Geometry check sheet. Reference: the model listing, model coordinates, mm. Face numbers are marked on the shaded views. A direction names the side the tool comes from. Give positions to 0.01 mm unless a question says otherwise; leave off trailing zeros. Loops run counter-clockwise (first coordinate to the right, second up) from the corner with the lowest first, then second, coordinate; pieces in that order, holes last. Notation, with made-up numbers: (-11, -33) -> (25, -33) arc R13 cw to (25, -28) -> close; hole circle Ø4 at (9, 36). An arc over 180 degrees is marked (long way). Answer as a JSON object with one key per item and string values.
from build123d import *

# Parameters (mm, degrees)
SKETCH1_W           = 36
SKETCH1_H           = 48
BOSS_EXTRUDE1_DEPTH = 1.5
SKETCH1_3_R         = 13
BOSS_EXTRUDE2_DEPTH = 8.5
SKETCH1_4_W         = 13
SKETCH1_4_H         = 13
BOSS_EXTRUDE3_DEPTH = 12
SKETCH1_5_R         = 1.6
CUT_EXTRUDE2_DEPTH  = 33.310988843


with BuildPart() as part:
    # Sketch1 → Boss-Extrude1 (new body)
    with BuildSketch(Plane(origin=(0, 0, 0), x_dir=(1, 0, 0), z_dir=(0, 1, 0))):
        Rectangle(SKETCH1_W, SKETCH1_H)
    extrude(amount=BOSS_EXTRUDE1_DEPTH)

    # Sketch1_3 → Boss-Extrude2 (add)
    with BuildSketch(Plane(origin=(0, 0, 0), x_dir=(1, 0, 0), z_dir=(0, 1, 0))):
        with Locations(Location((0, 6, 0), (0, 0, 90))):
            Circle(SKETCH1_3_R)
    extrude(amount=BOSS_EXTRUDE2_DEPTH)

    # Sketch1_4 → Boss-Extrude3 (add)
    with BuildSketch(Plane(origin=(0, 0, 0), x_dir=(1, 0, 0), z_dir=(0, 1, 0))):
        with Locations((-10, -12.5)):
            Rectangle(SKETCH1_4_W, SKETCH1_4_H)
    extrude(amount=BOSS_EXTRUDE3_DEPTH)

    # Sketch1_5 → Cut-Extrude2 (cut, through all)
    with BuildSketch(Plane(origin=(0, 0, 0), x_dir=(1, 0, 0), z_dir=(0, 1, 0))):
        with Locations(Location((0, -11.4, 0), (0, 0, 90))):
            Circle(SKETCH1_5_R)
    extrude(amount=CUT_EXTRUDE2_DEPTH, mode=Mode.SUBTRACT)


solid = part.part
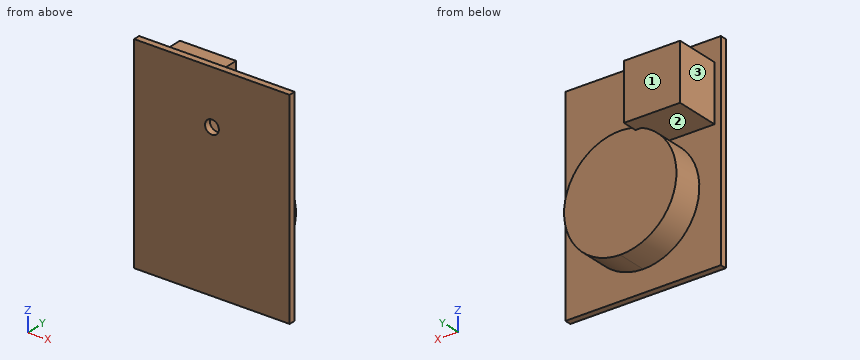
1) Material ranges on line 1 along X through (y, z) = (0.8, 11.4); line 2 along Y through (x, z) = (1.5, 9.5); line 3 along X through (y, z) = (8, -6), recorded low to high. Write a range as from..to.
Geometry check:
{"line 1": "x = -18..-1.6, 1.6..18", "line 2": "y = 0..1.5", "line 3": "x = -13..13"}
2) Tool access check on the marked faces 1, 2 and 3. Record the directions out of +Z, -Z, +X, -X, +Y, -Y that give a thin tool (end or side, any length) a straight path to the whole face; none if there is none.
Geometry check:
{"face 1": "+Z, -Z, +X, -X, +Y", "face 2": "-X, +Y", "face 3": "+Z, -Z, -X, +Y"}
3) Section check D-D on x = 12.5. Record the cut outline in (y, z).
Geometry check:
{"outline": "(0, -24) -> (1.5, -24) -> (1.5, -9.57) -> (8.5, -9.57) -> (8.5, -2.43) -> (1.5, -2.43) -> (1.5, 24) -> (0, 24) -> close"}
4) Depth check by flat-ended pin: P1, Ø3, axis at x = -10, y = 8, coming from the +Z side; P2, Ø1, axis at x = -6, z = -4.5, coming from the -Y side; P3, Ø13, axis at x = -2, z = -11.5, coming from the +Y side; P4, Ø5, axis at x = -8, y = 6.5, coming from the -Z side. Enter the tip coordinate at first touch or a pass-through.
Geometry check:
{"P1": "stops at z = 19", "P2": "stops at y = 0", "P3": "stops at y = 8.5", "P4": "stops at z = -17.78"}
5) Section check B-B on x = -0.5. Record the cut outline in (y, z).
Geometry check:
{"outline": "(0, -24) -> (1.5, -24) -> (1.5, -18.99) -> (8.5, -18.99) -> (8.5, 6.99) -> (1.5, 6.99) -> (1.5, 9.88) -> (0, 9.88) -> close; (0, 12.92) -> (1.5, 12.92) -> (1.5, 24) -> (0, 24) -> close"}
6) Section check C-C on z = 5.5. Record the cut outline in (x, y).
Geometry check:
{"outline": "(-18, 0) -> (18, 0) -> (18, 1.5) -> (6.06, 1.5) -> (6.06, 8.5) -> (-6.06, 8.5) -> (-6.06, 1.5) -> (-18, 1.5) -> close"}
7) Section check A-A on z = 11.4. Record the cut outline in (x, y), plus the area to 3 significant figures.
Geometry check:
{"outline": "(-18, 0) -> (-1.6, 0) -> (-1.6, 1.5) -> (-3.5, 1.5) -> (-3.5, 12) -> (-16.5, 12) -> (-16.5, 1.5) -> (-18, 1.5) -> close; (1.6, 0) -> (18, 0) -> (18, 1.5) -> (1.6, 1.5) -> close", "area": "186 mm2"}
